Check sheet for the modelled part. Datum: model origin and axes. Units: mm. A direction names the side the tool comes from. Round coordinates to 2 decimals unless told otherwise and drop trailing zeros. Order: outer loops, then holes, each group sorted by start corner. A loop starts at its lowest first (then second) coordinate and runs counter-clockwise, first axis right, second up.
Q1. Cross-section at A-A on y = 0. Record the cut outline in (x, z), then the cut area to 3 significant figures.
Q2. Cross-section at C-C on x = -5.75. Record the cut outline in (y, z).
Q3. Scan lines: probe 1 along Y at (x, z) = (-4.75, -7); probe 2 along Y at (x, z) = (0, 2); probe 3 along X at (y, z) = (-1.5, 2). Record each from-to range of solid material in increasing order.
Q4. Cross-section at B-B on z = -7.5. Record the cut outline in (x, y).
Q5. Set-up check for faces 4 (the flat face through (0, 9.5, -1)), 5 (the flat face through (0, 0, 3.5)), 6 (the flat face through (7.5, 0, 2)), 7 (the flat face through (0, -7.7, -4)), 8 (the flat face through (1, 5.9, -6)): record each of +Z, -Z, +X, -X, +Y, -Y from which the full face is reachable in a straight line by a thin tool's end or side.
Q6. Cross-section at D-D on z = 1.5. Record the cut outline in (x, y), then the cut area to 3 significant figures.
Q7. Mould release check, pull along X, two halves, no side actions. Record for faces 1 (the flat face through (-7.5, 0, -1)), 2 (the flat face through (0.721, -6.813, -4.383)), 3 (the flat face through (1, -5.9, -5)): +X half, -X half, draft (parallel to the pull), parting line (faces both ways), or undercut.
Q8. Depth check by flat-ended pin: P1, Ø3, axis at y = 6.5, z = -6, coming from the -X side; P2, Ø7, axis at x = 0, y = 0, coming from the -Z side; P3, Ø1.8, axis at y = 3, z = 1.5, coming from the +X side. Enter the tip coordinate at first touch or a pass-through.
from build123d import *

# Parameters (mm, degrees)
SKIZZE1_W                       = 15
SKIZZE1_H                       = 19
AUFSATZ_LINEAR_AUSTRAGEN1_DEPTH = 3
AUFSATZ_LINEAR_AUSTRAGEN2_DEPTH = 19
SKIZZE5_R                       = 3
SCHNITT_LINEAR_AUSTRAGEN1_DEPTH = 3
SKIZZE6_W                       = 15
SKIZZE6_H                       = 19
AUFSATZ_LINEAR_AUSTRAGEN3_DEPTH = 0.5
SKIZZE7_W                       = 15.962666587
SKIZZE7_H                       = 1.8
AUFSATZ_LINEAR_AUSTRAGEN4_DEPTH = 3.6
AUFSATZ_LINEAR_AUSTRAGEN5_DEPTH = 1.8
AUFSATZ_LINEAR_AUSTRAGEN6_DEPTH = 1.8


with BuildPart() as part:
    # Skizze1 → Aufsatz-Linear austragen1 (new body)
    with BuildSketch(Plane.XY):
        Rectangle(SKIZZE1_W, SKIZZE1_H)
    extrude(amount=AUFSATZ_LINEAR_AUSTRAGEN1_DEPTH)

    # Skizze3 → Aufsatz-Linear austragen2 (add)
    with BuildSketch(Plane(origin=(0, 9.5, 0), x_dir=(1, 0, 0), z_dir=(0, 1, 0))):
        Polygon((-7.5, 0), (-7.5, 5.459553514), (7.5, 0), align=None)
    extrude(amount=-AUFSATZ_LINEAR_AUSTRAGEN2_DEPTH)

    # Skizze5 → Schnitt-Linear austragen1 (cut)
    with BuildSketch(Plane.XY.offset(3)):
        Circle(SKIZZE5_R)
    extrude(amount=-SCHNITT_LINEAR_AUSTRAGEN1_DEPTH, mode=Mode.SUBTRACT)

    # Skizze6 → Aufsatz-Linear austragen3 (add)
    with BuildSketch(Plane.XY.offset(3)):
        Rectangle(SKIZZE6_W, SKIZZE6_H)
    extrude(amount=AUFSATZ_LINEAR_AUSTRAGEN3_DEPTH)

    # Skizze7 → Aufsatz-Linear austragen4 (add)
    with BuildSketch(Plane(origin=(0.877333338, 0, -2.410453536), x_dir=(-0.939692621, 0, -0.342020143), z_dir=(0.342020143, 0, -0.939692621))):
        with Locations((0.933638638, 8.6)):
            Rectangle(SKIZZE7_W, SKIZZE7_H)
        with Locations((0.933638638, -8.6)):
            Rectangle(SKIZZE7_W, SKIZZE7_H)
    extrude(amount=AUFSATZ_LINEAR_AUSTRAGEN4_DEPTH)

    # Skizze10 → Aufsatz-Linear austragen5 (add)
    with BuildSketch(Plane.XZ.offset(-7.7)):
        Polygon((8.731272516, -3.382893435), (8.115636258, -1.691446717), (-6.884363742, -7.151000231), (-6.268727484, -8.842446949), align=None)
    extrude(amount=AUFSATZ_LINEAR_AUSTRAGEN5_DEPTH)

    # Skizze9 → Aufsatz-Linear austragen6 (add)
    with BuildSketch(Plane(origin=(0, -7.7, 0), x_dir=(1, 0, 0), z_dir=(0, 1, 0))):
        Polygon((8.115636258, 1.691446717), (-6.884363742, 7.151000231), (-6.268727484, 8.842446949), (8.731272516, 3.382893435), align=None)
    extrude(amount=AUFSATZ_LINEAR_AUSTRAGEN6_DEPTH)


solid = part.part
Results found:
1. outline: (-7.5, -5.46) - (7.5, 0) - (7.5, 3.5) - (-7.5, 3.5) - close; hole (-3, 0) - (3, 0) - (3, 3) - (-3, 3) - close
1. area: 75.4 mm2
2. outline: (-9.5, -8.65) - (-5.9, -8.65) - (-5.9, -6.74) - (-7.7, -6.74) - (-7.7, -4.82) - (7.7, -4.82) - (7.7, -6.74) - (5.9, -6.74) - (5.9, -8.65) - (9.5, -8.65) - (9.5, 3.5) - (-9.5, 3.5) - close
3. probe 1: y = -9.5 to -5.9, 5.9 to 9.5
3. probe 2: y = -9.5 to -3, 3 to 9.5
3. probe 3: x = -7.5 to -2.6, 2.6 to 7.5
4. outline: (-6.76, -9.5) - (-2.58, -9.5) - (-2.58, -5.9) - (-6.76, -5.9) - close; (-6.76, 5.9) - (-2.58, 5.9) - (-2.58, 9.5) - (-6.76, 9.5) - close
5. face 4: +Z, -Z, +X, -X, +Y
5. face 5: +Z, +X, -X, +Y, -Y
5. face 6: +Z, +X, +Y, -Y
5. face 7: none
5. face 8: -Z, +X
6. outline: (-7.5, -9.5) - (7.5, -9.5) - (7.5, 9.5) - (-7.5, 9.5) - close; hole circle Ø6 at (0, 0)
6. area: 257 mm2
7. face 1: -X half
7. face 2: undercut
7. face 3: draft
8. P1: stops at x = -7.5
8. P2: stops at z = -4
8. P3: stops at x = 7.5
